The listing builds one solid part. Answer for the finished solid, in the listing's coordinates (mm). Give positions to 0.01 mm unless a question says otherwise; leave off trailing zeros. Write each loop counter-clockwise with the first axis right and the second up, starting at its lowest first coordinate (ties: lowest second). Pieces come first, ordered by that corner, then holes. Notation, with made-up numbers: (-21, 60.5) - (-12, 60.5) arc R8 ccw to (-12, 71.5) - close; hole circle Ø1 at (43, -38). An arc over 180 degrees is marked (long way). Answer as CSV lines item,"result". Start each with the question number.
(1) Straight lines are drawn through the part: probe 1 along X at (y, z) = (-0.4, 15.5); probe 2 along Y at (x, z) = (-0.15, 41.5); probe 3 along X at (y, z) = (0.75, 29.5). For each, find the intervals that lie inside material, in ascending order.
(2) Find section A-A (z = 60.5). Write down the section's boundary in (x, y) (3 decimals), then the cut area to 3 significant figures.
(3) Each of these flat-tipped pins is pushed along its axis until it touches: pin 1 Ø2 at (y, z) = (-1.5, 70) entering from +X; pin 2 Ø1.5 at (x, z) = (1, 53.5) entering from -Y. Where does it stop, or does it pass through?
from build123d import *

# Parameters (mm, degrees)
SKETCH2_R           = 1.905
BOSS_EXTRUDE1_DEPTH = 86.36
CHAMFER1_SIZE       = 2.54
CHAMFER1_SIZE2      = 0.222221205
FILLET1_R           = 12.7
FILLET2_R           = 0.635


with BuildPart() as part:
    # Sketch2 → Boss-Extrude1 (new body)
    with BuildSketch(Plane.XY):
        Circle(SKETCH2_R)
    extrude(amount=BOSS_EXTRUDE1_DEPTH)

    # Chamfer1
    chamfer1_edges = [part.edges().sort_by_distance(p)[0] for p in [
        (-1.905, 0, 86.36),
    ]]
    chamfer1_side = [part.faces().sort_by_distance(p)[0] for p in [
        (-1.905, 0, 43.18),
    ]]
    chamfer(chamfer1_edges, length=CHAMFER1_SIZE, length2=CHAMFER1_SIZE2, reference=chamfer1_side[0])

    # Fillet1
    # the kernel refuses this fillet: 12.7 mm, written as the material it takes off along each edge
    with BuildSketch(Plane(origin=(0, 0, 83.82), x_dir=(1, 0, 0), z_dir=(0, -1, 0))) as fillet1_piece_1:
        with BuildLine():
            CenterArc((1.905 - FILLET1_R, -FILLET1_R * 0.0436609429085), FILLET1_R, 0, 5)
            Line((1.905 - FILLET1_R * 0.00380530190825, FILLET1_R * 0.0434947998391), (1.905, 0))
            Line((1.905, 0), (1.905, -FILLET1_R * 0.0436609429085))
        make_face()
    revolve(axis=Axis((0, 0, 83.82), (0, 0, 1)), mode=Mode.SUBTRACT)

    # Fillet2
    fillet2_edges = [part.edges().sort_by_distance(p)[0] for p in [
        (-1.682778795, 0, 86.36),
    ]]
    fillet(fillet2_edges, radius=FILLET2_R)


solid = part.part
Result set:
1,probe 1,"-1.86 to 1.86"
1,probe 2,"-1.9 to 1.9"
1,probe 3,"-1.75 to 1.75"
2,outline,"circle Ø3.81 at (0, 0)"
2,area,"11.4 mm^2"
3,pin 1,"x = 1.84"
3,pin 2,"y = -1.89"
